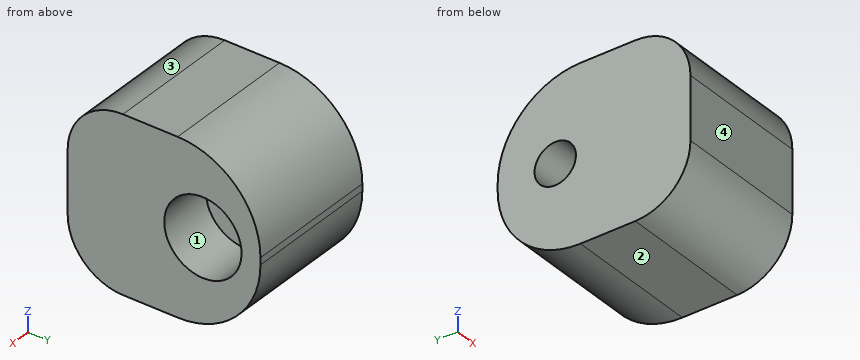
from build123d import *

# Parameters (mm, degrees)
SKETCH1_W           = 50.8
SKETCH1_H           = 9.525
BOSS_EXTRUDE1_DEPTH = 12.446
SKETCH6_R           = 1.905
CUT_EXTRUDE4_DEPTH  = 12.446
SKETCH7_R           = 3.556
CUT_EXTRUDE5_DEPTH  = 5.08
SKETCH8_W           = 38.1
SKETCH8_H           = 9.525
CUT_EXTRUDE6_DEPTH  = 12.446
FILLET2_R           = 2.54
CUT_EXTRUDE7_START  = -12.446
CUT_EXTRUDE7_DEPTH  = 12.446
FILLET4_R           = 5.08
SKETCH11_W          = 12.446
SKETCH11_H          = 9.525
BOSS_EXTRUDE2_DEPTH = 6.35
CUT_EXTRUDE8_START  = -12.446
SKETCH12_W          = 0.254
SKETCH12_H          = 9.525
CUT_EXTRUDE8_DEPTH  = 12.446
CUT_EXTRUDE9_START  = -12.446
CUT_EXTRUDE9_DEPTH  = 12.446
BOSS_EXTRUDE3_START = -12.446
BOSS_EXTRUDE3_DEPTH = 12.446
FILLET6_R           = 7.62
FILLET7_R           = 5.08


with BuildPart() as part:
    # Sketch1 → Boss-Extrude1 (new body)
    with BuildSketch(Plane.YZ):
        with Locations((-25.4, 4.7625)):
            Rectangle(SKETCH1_W, SKETCH1_H)
    extrude(amount=BOSS_EXTRUDE1_DEPTH)

    # Sketch6 → Cut-Extrude4 (cut)
    with BuildSketch(Plane.YZ.offset(12.446)):
        with Locations(Location((-44.45, 4.7625, 0), (0, 0, 270))):
            Circle(SKETCH6_R)
    extrude(amount=-CUT_EXTRUDE4_DEPTH, mode=Mode.SUBTRACT)

    # Sketch7 → Cut-Extrude5 (cut)
    with BuildSketch(Plane.YZ.offset(12.446)):
        with Locations(Location((-44.45, 4.7625, 0), (0, 0, 270))):
            Circle(SKETCH7_R)
    extrude(amount=-CUT_EXTRUDE5_DEPTH, mode=Mode.SUBTRACT)

    # Sketch8 → Cut-Extrude6 (cut)
    with BuildSketch(Plane.YZ.offset(12.446)):
        with Locations((-19.05, 4.7625)):
            Rectangle(SKETCH8_W, SKETCH8_H)
    extrude(amount=-CUT_EXTRUDE6_DEPTH, mode=Mode.SUBTRACT)

    # Fillet2
    fillet2_edges = [part.edges().sort_by_distance(p)[0] for p in [
        (6.223, -38.1, 0),
        (6.223, -38.1, 9.525),
    ]]
    fillet(fillet2_edges, radius=FILLET2_R)

    # Sketch9 → Cut-Extrude7 (cut)
    with BuildSketch(Plane.YZ.offset(12.446).offset(CUT_EXTRUDE7_START)):
        with BuildLine():
            Line((-40.64, 0), (-38.1, 2.54))
            ThreePointArc((-38.1, 2.54), (-38.843948776, 0.743948776), (-40.64, 0))
        make_face()
        with BuildLine():
            Line((-38.1, 6.985), (-40.64, 9.525))
            ThreePointArc((-40.64, 9.525), (-38.843948776, 8.781051224), (-38.1, 6.985))
        make_face()
    extrude(amount=CUT_EXTRUDE7_DEPTH, mode=Mode.SUBTRACT)

    # Fillet4
    fillet4_edges = [part.edges().sort_by_distance(p)[0] for p in [
        (6.223, -38.1, 2.54),
        (6.223, -38.1, 6.985),
    ]]
    fillet(fillet4_edges, radius=FILLET4_R)

    # Sketch11 → Boss-Extrude2 (add)
    with BuildSketch(Plane.XZ.offset(50.8)):
        with Locations((6.223, 4.7625)):
            Rectangle(SKETCH11_W, SKETCH11_H)
    extrude(amount=BOSS_EXTRUDE2_DEPTH)

    # Sketch12 → Cut-Extrude8 (cut)
    with BuildSketch(Plane.YZ.offset(12.446).offset(CUT_EXTRUDE8_START)):
        with Locations((-57.023, 4.7625)):
            Rectangle(SKETCH12_W, SKETCH12_H)
    extrude(amount=CUT_EXTRUDE8_DEPTH, mode=Mode.SUBTRACT)

    # Sketch13 → Cut-Extrude9 (cut)
    with BuildSketch(Plane.YZ.offset(12.446).offset(CUT_EXTRUDE9_START)):
        with BuildLine():
            Line((-39.153011094, 7.977528923), (-39.153011094, 1.547471077))
            ThreePointArc((-39.153011094, 1.547471077), (-38.370452015, 3.008769732), (-38.1, 4.644204897))
            Line((-38.1, 4.644204897), (-38.1, 4.880795103))
            ThreePointArc((-38.1, 4.880795103), (-38.370452015, 6.516230268), (-39.153011094, 7.977528923))
        make_face()
    extrude(amount=CUT_EXTRUDE9_DEPTH, mode=Mode.SUBTRACT)

    # Sketch14 → Boss-Extrude3 (add)
    with BuildSketch(Plane.YZ.offset(12.446).offset(BOSS_EXTRUDE3_START)):
        with BuildLine():
            Line((-39.153011094, 12.7), (-39.153011094, 7.977528923))
            ThreePointArc((-39.153011094, 7.977528923), (-39.362410998, 8.23227451), (-39.587897552, 8.472897552))
            Line((-39.587897552, 8.472897552), (-40.64, 9.525))
            Line((-40.64, 9.525), (-56.896, 9.525))
            Line((-56.896, 9.525), (-56.896, 12.7))
            Line((-56.896, 12.7), (-40.64, 12.7))
            Line((-40.64, 12.7), (-39.153011094, 12.7))
        make_face()
        with BuildLine():
            Line((-39.153011094, -3.175), (-40.64, -3.175))
            Line((-40.64, -3.175), (-56.896, -3.175))
            Line((-56.896, -3.175), (-56.896, 0))
            Line((-56.896, 0), (-40.64, 0))
            Line((-40.64, 0), (-39.587897552, 1.052102448))
            ThreePointArc((-39.587897552, 1.052102448), (-39.362410998, 1.29272549), (-39.153011094, 1.547471077))
            Line((-39.153011094, 1.547471077), (-39.153011094, -3.175))
        make_face()
    extrude(amount=BOSS_EXTRUDE3_DEPTH)

    # Fillet6
    fillet6_edges = [part.edges().sort_by_distance(p)[0] for p in [
        (6.223, -39.153011094, 12.7),
        (6.223, -39.153011094, -3.175),
    ]]
    fillet(fillet6_edges, radius=FILLET6_R)

    # Fillet7
    fillet7_edges = [part.edges().sort_by_distance(p)[0] for p in [
        (6.223, -56.896, 12.7),
        (6.223, -56.896, -3.175),
    ]]
    fillet(fillet7_edges, radius=FILLET7_R)


solid = part.part
Work out the finished part from the listing and answer in its coordinate system (mm). Face numbers are marked on the shaded views. Coordinates: 2 decimals unless noted, no trailing zeros. Loops run counter-clockwise (first coordinate to the right, second up) from the corner with the lowest first, then second, coordinate; pieces in that order, holes last. Notation, with made-up numbers: M 7.5,-35 L 18.5,-35 A10 ccw 18.5,-19 Z; hole C 77.25,29.25 d1. An arc over 180 degrees is marked long. Answer in a Markdown table with one row per item. Add a question column.
1. Find section C-C, the plane z = 4.75. Write down the section's boundary in (x, y), then the cut area to 3 significant figures.
2. Find section B-B, the plane y = -44.45. Write down the section's boundary in (x, z).
3. Consider L1, parallel to Y at x = 7.75, z = 4.75; L2, parallel to Y at x = 7.75, z = 2.75; L3, parallel to Z at x = 4.5, y = -45. Determine where each line is inside the solid, lowest interval first.
4. Flat-ended cylindrical pins translate along their axes: P1, Ø5, axis at x = 4.5, z = 0.5, coming from the +Y side; P2, Ø1.5, axis at x = 5.5, z = -0.5, coming from the +Y side; P3, Ø3, axis at y = -54.5, z = 1.5, coming from the -X side; P4, Ø1, axis at x = 6, y = -42.5, coming from the -Z side. Find the tip coordinate at first contact, or state that the pin passes through.
5. The mould has two halves that part along Z. Classify the marked faces 1, 2, 3 and 4: pulls with the +Z half, pulls with the -Z half, needs draft (parallel to the pull), parting line crosses it, or undercut.
Reported:
| question | item | result |
|---|---|---|
| 1 | outline | M 0,-56.9 L 12.45,-56.9 L 12.45,-48.01 L 7.37,-48.01 L 7.37,-46.35 L 0,-46.35 Z; M 0,-42.55 L 7.37,-42.55 L 7.37,-40.89 L 12.45,-40.89 L 12.45,-39.15 L 0,-39.15 Z |
| 1 | area | 157 mm^2 |
| 2 | outline | M 0,-2.81 L 12.45,-2.81 L 12.45,1.21 L 7.37,1.21 L 7.37,2.86 L 0,2.86 Z; M 0,6.67 L 7.37,6.67 L 7.37,8.32 L 12.45,8.32 L 12.45,12.34 L 0,12.34 Z |
| 3 | L1 | y = -56.9 to -48.01, -40.89 to -39.15 |
| 3 | L2 | y = -56.9 to -47.38, -41.52 to -39.34 |
| 3 | L3 | z = -2.97 to 2.94, 6.59 to 12.49 |
| 4 | P1 | stops at y = -39.29 |
| 4 | P2 | stops at y = -40.41 |
| 4 | P3 | stops at x = 0 |
| 4 | P4 | stops at z = -2.18 |
| 5 | face 1 | undercut |
| 5 | face 2 | pulls with the -Z half |
| 5 | face 3 | pulls with the +Z half |
| 5 | face 4 | needs draft |
